```python
from build123d import *

# Parameters (mm, degrees)
BASE_FLANGE1_DEPTH     = 0.91186
SKETCHED_BEND1_DEPTH   = 72.39
SKETCHED_BEND1_2_DEPTH = 72.39
EDGE_FLANGE1_DEPTH     = 29.038915496
EDGE_FLANGE2_DEPTH     = 29.038915496


# Read off the part's stored shape, not the designer's step: Sketched Bend1
# Sheet-metal steps are written as plain solids
with BuildPart() as part:
    # Sketch1 → Base-Flange1 (new body)
    with BuildSketch(Plane(origin=(0, 0, 0), x_dir=(1, 0, 0), z_dir=(0, 1, 0))):
        Polygon((0, 38.1), (22.86, 50.8), (49.53, 50.8), (72.39, 38.1), (72.39, 0), (0, 0), align=None)
    extrude(amount=-BASE_FLANGE1_DEPTH)

    # Sketched Bend1 outline → Sketched Bend1 (cut)
    with BuildSketch(Plane.YZ):
        with BuildLine():
            ThreePointArc((-0.91186, -31.75), (-0.670550858, -30.752615706), (0, -29.975848636))
            Line((0, -29.975848636), (0, 0))
            Line((0, 0), (-0.91186, 0))
            Line((-0.91186, 0), (-0.91186, -31.75))
        make_face()
    extrude(amount=SKETCHED_BEND1_DEPTH, mode=Mode.SUBTRACT)

    # Sketched Bend1 2 outline → Sketched Bend1 2 (add)
    with BuildSketch(Plane.YZ):
        with BuildLine():
            Line((30.308915496, -30.48), (30.308915496, -29.56814))
            Line((30.308915496, -29.56814), (1.27, -29.56814))
            ThreePointArc((1.27, -29.56814), (0.603080527, -29.672566131), (0, -29.975848636))
            Line((0, -29.975848636), (0, -31.75))
            ThreePointArc((0, -31.75), (0.371974388, -30.851974388), (1.27, -30.48))
            Line((1.27, -30.48), (30.308915496, -30.48))
        make_face()
    extrude(amount=SKETCHED_BEND1_2_DEPTH)

    # Edge-Flange1 section (across the edge) → Edge-Flange1 (add)
    with BuildSketch(Plane(origin=(-1.27, 1.27, -30.48), x_dir=(1, 0, 0), z_dir=(0, 1, 0))):
        with BuildLine():
            Line((-0.91186, 1.27), (-0.91186, 7.62))
            Line((-0.91186, 7.62), (0, 7.62))
            Line((0, 7.62), (0, 1.27))
            ThreePointArc((0, 1.27), (0.371974388, 0.371974388), (1.27, 0))
            Line((1.27, 0), (1.27, -0.91186))
            ThreePointArc((1.27, -0.91186), (-0.272808002, -0.272808002), (-0.91186, 1.27))
        make_face()
    extrude(amount=EDGE_FLANGE1_DEPTH)

    # Edge-Flange2 section (across the edge) → Edge-Flange2 (add)
    with BuildSketch(Plane(origin=(73.66, 30.308915496, -30.48), x_dir=(-1, 0, 0), z_dir=(0, -1, 0))):
        with BuildLine():
            Line((-0.91186, 1.27), (-0.91186, 7.62))
            Line((-0.91186, 7.62), (0, 7.62))
            Line((0, 7.62), (0, 1.27))
            ThreePointArc((0, 1.27), (0.371974388, 0.371974388), (1.27, 0))
            Line((1.27, 0), (1.27, -0.91186))
            ThreePointArc((1.27, -0.91186), (-0.272808002, -0.272808002), (-0.91186, 1.27))
        make_face()
    extrude(amount=EDGE_FLANGE2_DEPTH)


solid = part.part
```
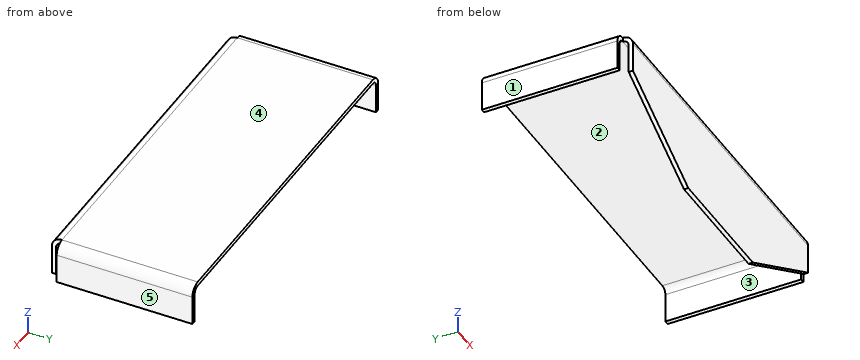
Work out the finished part from the listing and answer in its coordinate system (mm). Face numbers are marked on the shaded views. A direction names the side the tool comes from. Give positions to 0.01 mm unless a question says otherwise; leave off trailing zeros. Write each loop counter-clockwise with the first axis right and the second up, starting at its lowest first coordinate (ties: lowest second). Pieces come first, ordered by that corner, then holes.
(1) Flat-ended cylindrical pins translate along their axes: pin 1 Ø1.5 at (x, z) = (35, -45.5) entering from +Y; pin 2 Ø8 at (x, y) = (28, 9) entering from -Z; pin 3 Ø0.7 at (y, z) = (0.5, -33.5) entering from +X; pin 4 Ø0.7 at (x, z) = (73.5, -35.5) entering from -Y. Find the tip coordinate at first contact, or state that the pin passes through.
Final values:
pin 1: stops at y = 0
pin 2: stops at z = -30.48
pin 3: passes through
pin 4: stops at y = 1.27
(2) The mould has two halves that part along X. Classify the marked faces 3, 4 and 5: pulls with the +X half, pulls with the -X half, needs draft (parallel to the pull), parting line crosses it, or undercut.
Final values:
face 3: undercut
face 4: needs draft
face 5: pulls with the +X half
(3) The part is cut by section D-D on x = 9. Write down the section's boundary in (y, z), plus the area to 3 significant figures.
Final values:
outline: (-0.91, -43.1) - (0, -43.1) - (0, -31.75) arc R1.27 cw to (1.27, -30.48) - (30.31, -30.48) - (30.31, -29.57) - (1.27, -29.57) arc R2.18 ccw to (-0.91, -31.75) - close
area: 39.3 mm2
(4) Straight lines are drawn through the part: line 1 (X direction, y = 21, z = -36.5); line 2 (Z direction, x = 19, y = 26); line 3 (Y direction, x = 27.5, z = -37.25). For each, find the intervals that lie inside material, in ascending order.
Final values:
line 1: x = -2.18 to -1.27, 73.66 to 74.57
line 2: z = -30.48 to -29.57
line 3: y = -0.91 to 0
(5) The part is cut by section A-A on z = -36. Write down the section's boundary in (x, y), plus the area to 3 significant figures.
Final values:
outline: (-2.18, 1.27) - (-1.27, 1.27) - (-1.27, 30.31) - (-2.18, 30.31) - close; (0, -0.91) - (72.39, -0.91) - (72.39, 0) - (0, 0) - close; (73.66, 1.27) - (74.57, 1.27) - (74.57, 30.31) - (73.66, 30.31) - close
area: 119 mm2
(6) Which of the six approach directions +Z, -Z, +X, -X, +Y, -Y give full straight-line access (tool end or side, diameter ignored) to the marked faces 1 and 2?
Final values:
face 1: +Z, -Z, -X, +Y, -Y
face 2: -Z, +Y
(7) The part is cut by section B-B on x = 57. Write down the section's boundary in (y, z), plus the area to 3 significant figures.
Final values:
outline: (-0.91, -46.65) - (0, -46.65) - (0, -31.75) arc R1.27 cw to (1.27, -30.48) - (30.31, -30.48) - (30.31, -29.57) - (1.27, -29.57) arc R2.18 ccw to (-0.91, -31.75) - close
area: 42.5 mm2
(8) The part is cut by section C-C on y = 14. Write down the section's boundary in (x, z).
Final values:
outline: (-2.18, -38.1) - (-1.27, -38.1) - (-1.27, -31.75) arc R1.27 cw to (0, -30.48) - (72.39, -30.48) arc R1.27 cw to (73.66, -31.75) - (73.66, -38.1) - (74.57, -38.1) - (74.57, -31.75) arc R2.18 ccw to (72.39, -29.57) - (0, -29.57) arc R2.18 ccw to (-2.18, -31.75) - close
